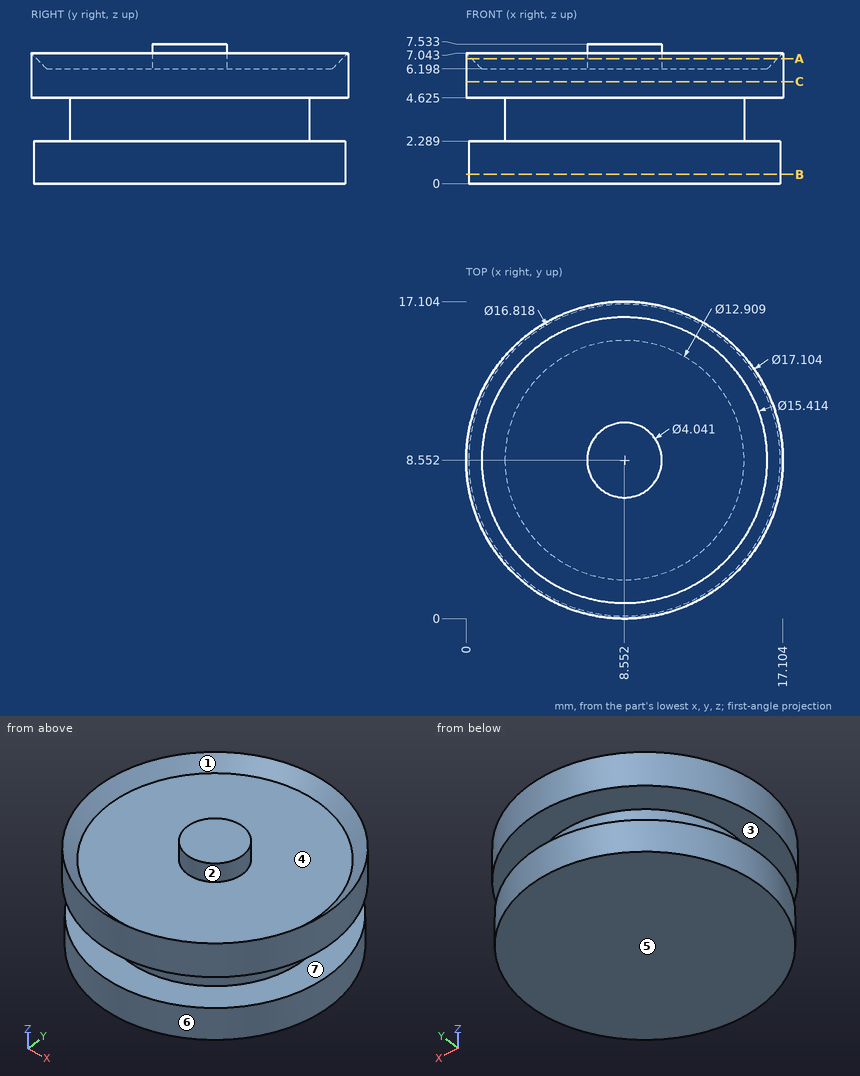
The drawing under review shows one solid part. Ordinate dimensions are in mm from its lowest x, y, z. A direction names the side the tool comes from. Coordinates: 2 decimals unless noted, no trailing zeros. Write each loop counter-clockwise with the first axis right and the second up, starting at its lowest first coordinate (ties: lowest second). Pieces come first, ordered by that corner, then holes. Notation, with made-up numbers: (49.5, -15.75) - (98.5, -15.75) arc R13 cw to (98.5, 1.25) - close; hole circle Ø8 at (-31, 2.25). An arc over 180 degrees is marked (long way). Put each result on its own line as item: value.
1. Add section C-C, the plane z = 5.5. Give the boundary of the cut face in (x, y) (1 decimal).
Values found:
outline: circle Ø17.1 at (8.6, 8.6)
2. Mouldability with a two-part tool opening along Z and no side actions: class the marked faces 1, 2 and 3 as released by +Z, released by -Z, zero draft, split by the parting line, or undercut.
Values found:
face 1: released by +Z
face 2: zero draft
face 3: undercut
3. Add section B-B, the plane z = 0.5. Give the boundary of the cut face in (x, y).
Values found:
outline: circle Ø16.82 at (8.55, 8.55)
4. Wall thickness on probe 1 along Z at (x, y) = (15.5, 6.75) (1 decimal); probe 2 along X at (y, z) = (9, 6.25) (1 decimal); probe 3 along Z at (x, y) = (14.75, 9.5): over which ranges is each line inside the solid? List them lowest first.
Values found:
probe 1: 0 to 2.3, 4.6 to 6.2
probe 2: 0 to 0.8, 6.6 to 10.5, 16.3 to 17.1
probe 3: 0 to 6.2
5. For pin 1 (2 mm diameter, centred on x = 11.5, y = 15, fed in from +Z); pin 2 (5 mm diameter, centred on x = 2, y = 12, fed in from -Z); pin 3 (3 mm diameter, centred on x = 4, z = 1.5, fed in from +Y); pin 4 (3 mm diameter, centred on y = 13, z = 3, fed in from -X), all flat-tipped, find the tip position at first contact; note any pin that passes through.
Values found:
pin 1: z = 6.58
pin 2: z = 0
pin 3: y = 16.39
pin 4: x = 0.75
6. Add section A-A, the plane z = 6.75. Give the boundary of the cut face in (x, y) (1 decimal).
Values found:
outline: circle Ø17.1 at (8.6, 8.6); circle Ø4 at (8.6, 8.6); hole circle Ø16.5 at (8.6, 8.6)
7. Machinability: for the marked faces 4, 5, 6 and 7, which of the approach directions +Z, -Z, +X, -X, +Y, -Y give a long, thin tool a straight path to every point of the face, cutting with its end or side? Answer none if there is none.
Values found:
face 4: +Z
face 5: -Z, +X, -X, +Y, -Y
face 6: -Z
face 7: none
